Read the model definition and answer for the solid it produces. Units are mm, in the model's axes. A direction names the side the tool comes from. Round coordinates to 2 decimals unless told otherwise and drop trailing zeros. Loops run counter-clockwise (first coordinate to the right, second up) from the corner with the lowest first, then second, coordinate; pieces in that order, holes last. Notation, with made-up numbers: (20.5, 31.25) -> (25.5, 31.25) arc R19 cw to (25.5, 68.25) -> close; hole circle Ø3 at (38.25, -3.5). An arc over 180 degrees is marked (long way). Put each result on its own line as item: value.
from build123d import *

# Parameters (mm, degrees)
SKETCH1_W           = 22.5
SKETCH1_H           = 12.15
BOSS_EXTRUDE1_DEPTH = 22.5
SKETCH2_W           = 12.15
SKETCH2_H           = 2.55
BOSS_EXTRUDE2_DEPTH = 5
SKETCH3_R           = 1
CUT_EXTRUDE1_DEPTH  = 2.55
SKETCH4_R           = 2.25
BOSS_EXTRUDE3_DEPTH = 10


with BuildPart() as part:
    # Sketch1 → Boss-Extrude1 (new body)
    with BuildSketch(Plane(origin=(0, 0, 0), x_dir=(1, 0, 0), z_dir=(0, 1, 0))):
        Rectangle(SKETCH1_W, SKETCH1_H)
    extrude(amount=BOSS_EXTRUDE1_DEPTH)

    # Sketch2 → Boss-Extrude2 (add)
    with BuildSketch(Plane(origin=(11.25, 0, 0), x_dir=(0, 0, -1), z_dir=(1, 0, 0))):
        with Locations((0, 19.425)):
            Rectangle(SKETCH2_W, SKETCH2_H)
    boss_extrude2 = extrude(amount=BOSS_EXTRUDE2_DEPTH)

    # Sketch3 → Cut-Extrude1 (cut)
    with BuildSketch(Plane(origin=(0, 20.7, 0), x_dir=(1, 0, 0), z_dir=(0, 1, 0))):
        with Locations(Location((14.25, 0, 0), (0, 0, 270))):
            Circle(SKETCH3_R)
    cut_extrude1 = extrude(amount=-CUT_EXTRUDE1_DEPTH, mode=Mode.SUBTRACT)

    # Mirror1: Boss-Extrude2, Cut-Extrude1 across plane
    add(boss_extrude2.mirror(Plane(origin=(0, 0, 0), x_dir=(0, 0, 1), z_dir=(1, 0, 0))))
    add(cut_extrude1.mirror(Plane(origin=(0, 0, 0), x_dir=(0, 0, 1), z_dir=(1, 0, 0))), mode=Mode.SUBTRACT)

    # Sketch4 → Boss-Extrude3 (add)
    with BuildSketch(Plane(origin=(0, 22.5, 0), x_dir=(1, 0, 0), z_dir=(0, 1, 0))):
        with Locations(Location((6.25, 0, 0), (0, 0, 270))):
            Circle(SKETCH4_R)
    extrude(amount=BOSS_EXTRUDE3_DEPTH)


solid = part.part
Item 1: Find the intervals of material crossed by line 1 along X through (y, z) = (19.5, 0); line 2 along Z through (x, y) = (-14.25, 18.8) (3 decimals); line 3 along Y through (x, z) = (8, 4), in increasing order.
Derived:
line 1: x = -16.25 to -15.25, -13.25 to 13.25, 15.25 to 16.25
line 2: z = -6.075 to -1, 1 to 6.075
line 3: y = 0 to 22.5
Item 2: For a pull along Z with two mould halves and no side action, classify faces 4 (the cylindrical face through (6.926, 27.43, 2.146)), 5 (the flat face through (16.25, 19, 0)), 6 (the cylindrical face through (-13.274, 19.443, -0.217)), 7 (the flat face through (0, 11, -6.075)) as pulls with the +Z half, pulls with the -Z half, needs draft (parallel to the pull), parting line crosses it, or undercut.
Derived:
face 4: parting line crosses it
face 5: needs draft
face 6: undercut
face 7: pulls with the -Z half
Item 3: The part is cut by section C-C (x = 6.25). Determine the outline of the cut face in (y, z) (3 decimals), then the cut area to 3 significant figures.
Derived:
outline: (0, -6.075) -> (22.5, -6.075) -> (22.5, -2.25) -> (32.5, -2.25) -> (32.5, 2.25) -> (22.5, 2.25) -> (22.5, 6.075) -> (0, 6.075) -> close
area: 318 mm^2
Item 4: Flat-ended cylindrical pins translate along their axes: pin 1 Ø2.5 at (x, z) = (14.25, 0) entering from +Y; pin 2 Ø5.5 at (x, z) = (-13, 2) entering from +Y; pin 3 Ø2 at (y, z) = (15.5, 0) entering from +X. Find the tip coordinate at first contact, or state that the pin passes through.
Derived:
pin 1: stops at y = 20.7
pin 2: stops at y = 22.5
pin 3: stops at x = 11.25
Item 5: The part is cut by section D-D (z = 4). Determine the outline of the cut face in (x, y).
Derived:
outline: (-16.25, 18.15) -> (-11.25, 18.15) -> (-11.25, 0) -> (11.25, 0) -> (11.25, 18.15) -> (16.25, 18.15) -> (16.25, 20.7) -> (11.25, 20.7) -> (11.25, 22.5) -> (-11.25, 22.5) -> (-11.25, 20.7) -> (-16.25, 20.7) -> close
Item 6: The part is cut by section B-B (z = 0). Determine the outline of the cut face in (x, y), then the cut area to 3 significant figures.
Derived:
outline: (-16.25, 18.15) -> (-15.25, 18.15) -> (-15.25, 20.7) -> (-16.25, 20.7) -> close; (-13.25, 18.15) -> (-11.25, 18.15) -> (-11.25, 0) -> (11.25, 0) -> (11.25, 18.15) -> (13.25, 18.15) -> (13.25, 20.7) -> (11.25, 20.7) -> (11.25, 22.5) -> (8.5, 22.5) -> (8.5, 32.5) -> (4, 32.5) -> (4, 22.5) -> (-11.25, 22.5) -> (-11.25, 20.7) -> (-13.25, 20.7) -> close; (15.25, 18.15) -> (16.25, 18.15) -> (16.25, 20.7) -> (15.25, 20.7) -> close
area: 567 mm^2
Item 7: The part is cut by section A-A (x = -14.25). Determine the outline of the cut face in (y, z) (3 decimals), then the cut area to 3 significant figures.
Derived:
outline: (18.15, -6.075) -> (20.7, -6.075) -> (20.7, -1) -> (18.15, -1) -> close; (18.15, 1) -> (20.7, 1) -> (20.7, 6.075) -> (18.15, 6.075) -> close
area: 25.9 mm^2
Item 8: Which of the six approach directions +Z, -Z, +X, -X, +Y, -Y give full straight-line access (tool end or side, diameter ignored) to faces 1 (the flat face through (13, 20.7, 0)), 2 (the flat face through (-11.25, 9, 0)), 3 (the flat face through (-11.25, 22, 0))?
Derived:
face 1: +Z, -Z, +X, +Y
face 2: +Z, -Z, -X, -Y
face 3: +Z, -Z, -X, +Y
